Part model, mm, in its own coordinate system. A direction names the side the tool comes from. Coordinates: 2 decimals unless noted, no trailing zeros. Write each loop counter-clockwise with the first axis right and the second up, starting at its lowest first coordinate (ties: lowest second). Pieces come first, ordered by that corner, then holes. Notation, with made-up numbers: M -38.5,-35.75 L -29.5,-35.75 A16 ccw -29.5,-21.75 Z; hole C 84,45 d11. An arc over 180 degrees is marked long. Use a Markdown table: item, result. Add a question column.
Q1. Wall check: L1, parallel to Z at x = -5.25, y = 25; L2, parallel to Z at x = 63, y = -14.5. Give the ranges that are in metal, low to high. Write a range as from..to.
Q2. Slice it at B-B on y = 25. Write the cut outline in (x, z).
Q3. Tool access for faces 1 (the cylindrical face through (-4.93, 67.419, 73.794)), 2 (the flat face through (41, -5, 24)), 3 (the flat face through (79, -18, 0)): list every direction of +Z, -Z, +X, -X, +Y, -Y with a clear straight run to the whole face (end or side of a thin tool).
Q4. Mould opens along Z. For faces 4 (the cylindrical face through (-4.93, -62.581, 73.794)), 5 (the flat face through (41, 5, 24)), 6 (the flat face through (76.05, -0.07, 41.905)) say: released by +Z, released by -Z, zero draft, split by the parting line, or undercut.
Q5. Slice it at C-C on x = 40. Write the cut outline in (y, z), then the cut area to 3 significant figures.
Q6. Pin check, flat tips, straight feed: pin 1 Ø3 at (y, z) = (-52, 52) entering from +X; pin 2 Ø4 at (x, y) = (52, -3.5) entering from +Z; pin 3 Ø4 at (x, z) = (24, 68) entering from +Y; pin 4 Ø5.5 at (y, z) = (-25, 70) entering from +X. Stop position of each tip, or through.
Q7. Slice it at A-A on y = -50. Write the cut outline in (x, z).
Q8. Slice it at D-D on y = 2. Write the cut outline in (x, z), then the cut area to 4 significant figures.
from build123d import *

# Parameters (mm, degrees)
F1_DEPTH      = 75
F1_DEPTH_BACK = 75
F3_DEPTH      = 5
F3_DEPTH_BACK = 5
F4_R          = 4.5
F5_DEPTH      = 10
F6_R          = 12.5
F7_DEPTH      = 10


with BuildPart() as f1:
    # F0 (on Front) → F1 (new body, two sides)
    with BuildSketch(Plane.XZ) as f1_sk:
        Polygon((0, 90), (-10, 90), (-10, -10), (155, -10), (155, 0), (0, 0), align=None)
    extrude(amount=F1_DEPTH)
    extrude(f1_sk.sketch, amount=-F1_DEPTH_BACK)

    # F2 (on Front) → F3 (join, two sides)
    with BuildSketch(Plane.XZ) as f3_sk:
        Polygon((150, 0), (0, 85), (0, 0), align=None)
    extrude(amount=F3_DEPTH)
    extrude(f3_sk.sketch, amount=-F3_DEPTH_BACK)

    # F4 (on Right) → F5 (cut, through all)
    with BuildSketch(Plane.YZ):
        with Locations((-65, 70)):
            Circle(F4_R)
        with Locations((-25, 70)):
            Circle(F4_R)
        with Locations((25, 70)):
            Circle(F4_R)
        with Locations((65, 70)):
            Circle(F4_R)
    extrude(amount=-F5_DEPTH, mode=Mode.SUBTRACT)

    # F6 (on Top) → F7 (cut, through all)
    with BuildSketch(Plane.XY):
        with Locations((40, 50)):
            Circle(F6_R)
        with Locations((115, 50)):
            Circle(F6_R)
        with Locations((115, -50)):
            Circle(F6_R)
        with Locations((40, -50)):
            Circle(F6_R)
    extrude(amount=-F7_DEPTH, mode=Mode.SUBTRACT)


solid = f1.part
Recorded:
| question | item | result |
|---|---|---|
| 1 | L1 | -10..65.5, 74.5..90 |
| 1 | L2 | -10..0 |
| 2 | outline | M -10,-10 L 155,-10 L 155,0 L 0,0 L 0,65.5 L -10,65.5 Z; M -10,74.5 L 0,74.5 L 0,90 L -10,90 Z |
| 3 | face 1 | +X, -X |
| 3 | face 2 | +Z, +X, -Y |
| 3 | face 3 | +Z, +X |
| 4 | face 4 | undercut |
| 4 | face 5 | zero draft |
| 4 | face 6 | released by +Z |
| 5 | outline | M -75,-10 L -62.5,-10 L -62.5,0 L -75,0 Z; M -37.5,-10 L 37.5,-10 L 37.5,0 L 5,0 L 5,62.33 L -5,62.33 L -5,0 L -37.5,0 Z; M 62.5,-10 L 75,-10 L 75,0 L 62.5,0 Z |
| 5 | area | 1,620 mm² |
| 6 | pin 1 | x = 0 |
| 6 | pin 2 | z = 56.67 |
| 6 | pin 3 | y = 5 |
| 6 | pin 4 | through |
| 7 | outline | M -10,-10 L 27.5,-10 L 27.5,0 L 0,0 L 0,90 L -10,90 Z; M 52.5,-10 L 102.5,-10 L 102.5,0 L 52.5,0 Z; M 127.5,-10 L 155,-10 L 155,0 L 127.5,0 Z |
| 8 | outline | M -10,-10 L 155,-10 L 155,0 L 150,0 L 0,85 L 0,90 L -10,90 Z |
| 8 | area | 8,925 mm² |
